```python
from build123d import *

# Parameters (mm, degrees)
F0_R     = 3.5
F1_DEPTH = 4
F2_R     = 2
F3_DEPTH = 10
F5_DEPTH = 2


with BuildPart() as f1:
    # F0 (on Front) → F1 (new body)
    with BuildSketch(Plane.XZ):
        Circle(F0_R)
    extrude(amount=F1_DEPTH)

    # F2 (on face) → F3 (join)
    with BuildSketch(Plane(origin=(0, 0, 0), x_dir=(-1, 0, 0), z_dir=(0, 1, 0))):
        Circle(F2_R)
    extrude(amount=F3_DEPTH)

    # F4 (on face) → F5 (cut)
    with BuildSketch(Plane.XZ.offset(4)):
        Polygon((0.866025, 1.5), (-0.866025, 1.5), (-1.732051, 0), (-0.866025, -1.5), (0.866025, -1.5), (1.732051, 0), align=None)
    extrude(amount=-F5_DEPTH, mode=Mode.SUBTRACT)


solid = f1.part
```
Geometry check sheet. Reference: the model listing, model coordinates, mm. A direction names the side the tool comes from. Round coordinates to 2 decimals unless told otherwise and drop trailing zeros. Order: outer loops, then holes, each group sorted by start corner. A loop starts at its lowest first (then second) coordinate and runs counter-clockwise, first axis right, second up. Notation, with made-up numbers: (14, 10.5) - (48, 10.5) arc R29 ccw to (48, 42.5) - close; hole circle Ø7 at (88.25, -8). An arc over 180 degrees is marked (long way). Use a Markdown table: item, result. Add a question column.
1) Gauge pin test, flat ends, axial feed: P1, Ø4, axis at y = 0.5, z = -2.5, coming from the -X side; P2, Ø1, axis at x = -1, y = 7, coming from the +Z side; P3, Ø2, axis at y = 1.5, z = -1, coming from the -X side. Record the tip position at first contact, or that the pin passes through.
2) Section check D-D (y = 1.75). Record the cut outline in (x, z), then the cut area to 3 significant figures.
3) Section check A-A (y = -2.25). Record the cut outline in (x, z).
4) Section check B-B (x = 0). Record the cut outline in (y, z), then the cut area to 3 significant figures.
5) Section check C-C (z = 0.75). Record the cut outline in (x, y), then the cut area to 3 significant figures.
6) Set-up check for faces 5 (the flat face through (2, 0, -2)), 6 (the flat face through (0, -3, 1.5)), 7 (the cylindrical face through (3.233, -1.972, -1.341)): record each of +Z, -Z, +X, -X, +Y, -Y from which the full face is reachable in a straight line by a thin tool's end or side.
7) Thickness scan on line 1 along Y through (x, z) = (2, 1); line 2 along Y through (x, z) = (0.75, -1); line 3 along Z through (x, y) = (-1.5, -2.75). Record the ranges inside material, lowest first.
8) Mould release check, pull along Z, two halves, no side actions. Record for faces 1 (the flat face through (1.305, -3.014, 0.74)), 2 (the cylindrical face through (0, 5, -2)), 3 (the flat face through (-1.293, -3.014, 0.76)), 4 (the flat face through (0, 10, 0)): released by +Z, released by -Z, zero draft, split by the parting line, or undercut.
Established:
| question | item | result |
|---|---|---|
| 1 | P1 | x = -3.45 |
| 1 | P2 | z = 1.94 |
| 1 | P3 | x = -2 |
| 2 | outline | circle Ø4 at (0, 0) |
| 2 | area | 12.6 mm2 |
| 3 | outline | circle Ø7 at (0, 0); hole (-1.73, 0) - (-0.87, -1.5) - (0.87, -1.5) - (1.73, 0) - (0.87, 1.5) - (-0.87, 1.5) - close |
| 4 | outline | (-4, -3.5) - (0, -3.5) - (0, -2) - (10, -2) - (10, 2) - (0, 2) - (0, 3.5) - (-4, 3.5) - (-4, 1.5) - (-2, 1.5) - (-2, -1.5) - (-4, -1.5) - close |
| 4 | area | 62.0 mm2 |
| 5 | outline | (-3.42, -4) - (-1.3, -4) - (-1.3, -2) - (1.3, -2) - (1.3, -4) - (3.42, -4) - (3.42, 0) - (1.85, 0) - (1.85, 10) - (-1.85, 10) - (-1.85, 0) - (-3.42, 0) - close |
| 5 | area | 59.2 mm2 |
| 6 | face 5 | +Y |
| 6 | face 6 | -Y |
| 6 | face 7 | +Y, -Y |
| 7 | line 1 | -4 to 0 |
| 7 | line 2 | -2 to 10 |
| 7 | line 3 | -3.16 to -0.4, 0.4 to 3.16 |
| 8 | face 1 | undercut |
| 8 | face 2 | split by the parting line |
| 8 | face 3 | undercut |
| 8 | face 4 | zero draft |
